Verification items for this drawing (mm, ordinates from the low corner). A direction names the side the tool comes from. Give positions to 0.01 mm unless a question says otherwise; leave off trailing zeros. Write each loop counter-clockwise with the first axis right and the second up, starting at its lowest first coordinate (ties: lowest second). Pieces come first, ordered by that corner, then holes. Notation, with made-up numbers: (35, 5) -> (58, 5) arc R9 ccw to (58, 15) -> close; hole circle Ø10 at (-21.75, 12.25). An arc over 180 degrees is marked (long way). Answer as a JSON object with one key per item and string values.
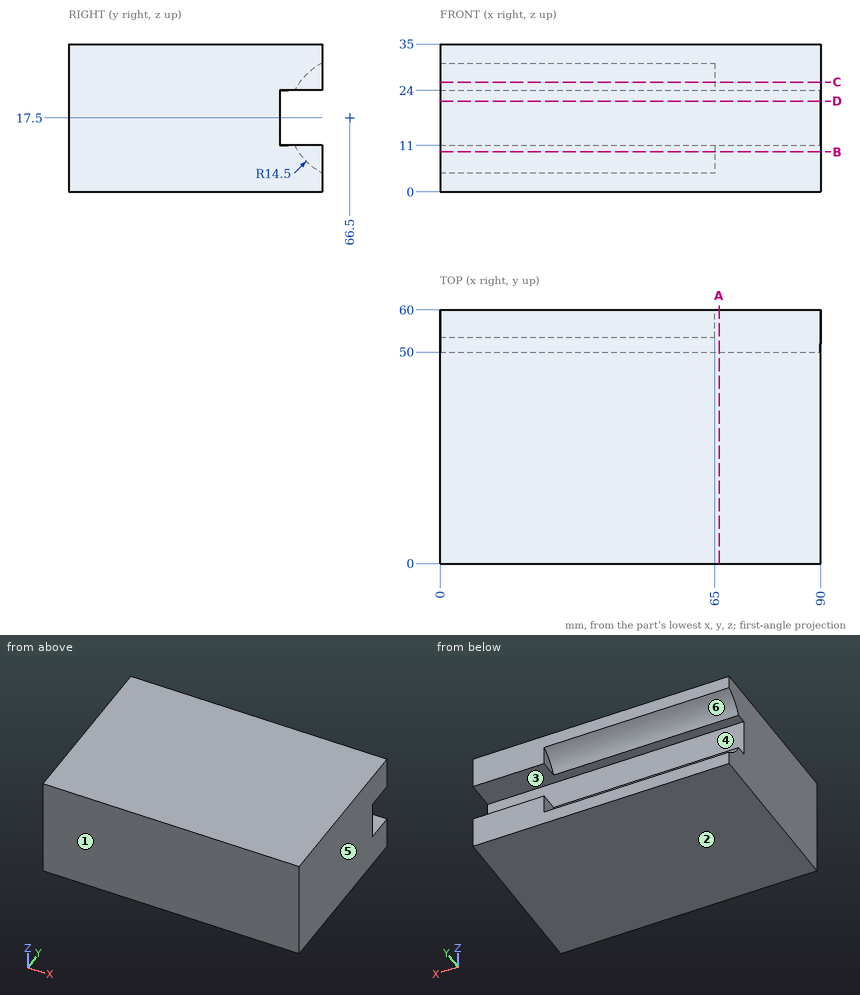
1. Sectioned sample at A-A, the plane x = 66. Enter the section's corners in (y, z).
Determined:
{"outline": "(0, 0) -> (60, 0) -> (60, 11) -> (50, 11) -> (50, 24) -> (60, 24) -> (60, 35) -> (0, 35) -> close"}
2. Access from +Z, -Z, +X, -X, +Y, -Y to the whole of each face (thin tool, end or side, straight path). Record for the marked faces 4, 5 and 6.
Determined:
{"face 4": "+X, -X, +Y", "face 5": "+Z, -Z, +X, +Y, -Y", "face 6": "-X, +Y"}
3. Sectioned sample at D-D, the plane z = 21.5. Enter the section's corners in (x, y).
Determined:
{"outline": "(0, 0) -> (90, 0) -> (90, 50) -> (0, 50) -> close"}
4. Scan lines: L1, parallel to Z at x = 77.5, y = 53; L2, parallel to Y at x = 24, z = 11.5; L3, parallel to X at y = 56.5, z = 8. Record each from-to range of solid material in increasing order. Write a range as [from, to].
Determined:
{"L1": "[0, 11], [24, 35]", "L2": "[0, 50]", "L3": "[65, 90]"}
5. Sectioned sample at B-B, the plane z = 9.5. Enter the section's corners in (x, y), plus the area to 3 significant figures.
Determined:
{"outline": "(0, 0) -> (90, 0) -> (90, 60) -> (65, 60) -> (65, 54.41) -> (0, 54.41) -> close", "area": "5,040 mm^2"}
6. Go/stop test with flat-tipped pins: P1, Ø6, axis at x = 34.5, z = 18.5, coming from the +Y side; P2, Ø5, axis at x = 48, z = 25.5, coming from the +Y side. Record where each tip stops, or that it passes through.
Determined:
{"P1": "y = 50", "P2": "y = 56.5"}
7. Sectioned sample at C-C, the plane z = 26. Enter the section's corners in (x, y).
Determined:
{"outline": "(0, 0) -> (90, 0) -> (90, 60) -> (65, 60) -> (65, 54.75) -> (0, 54.75) -> close"}
8. Mould release check, pull along Z, two halves, no side actions. Record for the marked faces 1, 2 and 3: released by +Z, released by -Z, zero draft, split by the parting line, or undercut.
Determined:
{"face 1": "zero draft", "face 2": "released by -Z", "face 3": "undercut"}
